from build123d import *

# Parameters (mm, degrees)
F1_DEPTH = 76.2
F2_R     = 12.7
F3_DEPTH = 25.4
F5_DEPTH = 25.4
F6_R     = 38.1
F7_R     = 38.1
F8_R     = 19.629033
F8_R_2   = 12.7
F9_DEPTH = 6.35


with BuildPart() as f1:
    # F0 (on Front) → F1 (new body, symmetric)
    with BuildSketch(Plane.XZ):
        Polygon((-76.2, 0), (0, 0), (0, 152.4), (-25.4, 152.4), (-25.4, 25.4), (-76.2, 25.4), align=None)
    extrude(amount=F1_DEPTH, both=True)

    # F2 (on face) → F3 (cut)
    with BuildSketch(Plane.YZ):
        with Locations((0, 101.6)):
            Circle(F2_R)
    extrude(amount=-F3_DEPTH, mode=Mode.SUBTRACT)

    # F4 (on face) → F5 (cut)
    with BuildSketch(Plane(origin=(0, 0, 0), x_dir=(1, 0, 0), z_dir=(0, 0, -1))):
        with BuildLine():
            ThreePointArc((-63.500749, -6.349625), (-69.781771, 0), (-63.500749, 6.349625))
            Line((-63.500749, 6.349625), (-76.2, 6.211669))
            Line((-76.2, 6.211669), (-76.2, -6.211669))
            Line((-76.2, -6.211669), (-63.500749, -6.349625))
        make_face()
        with BuildLine():
            ThreePointArc((-63.500749, -6.349625), (-58.966097, -4.51445), (-57.081771, 0))
            ThreePointArc((-57.081771, 0), (-58.966097, 4.51445), (-63.500749, 6.349625))
            ThreePointArc((-63.500749, 6.349625), (-69.781771, 0), (-63.500749, -6.349625))
        make_face()
    extrude(amount=-F5_DEPTH, mode=Mode.SUBTRACT)

    # F6
    f6_edges = [f1.edges().sort_by_distance(p)[0] for p in [
        (-12.7, -76.2, 152.4),
    ]]
    fillet(f6_edges, radius=F6_R)

    # F7
    f7_edges = [f1.edges().sort_by_distance(p)[0] for p in [
        (-12.7, 76.2, 152.4),
    ]]
    fillet(f7_edges, radius=F7_R)

    # F8 (on face) → F9 (cut)
    with BuildSketch(Plane(origin=(-25.4, 0, 0), x_dir=(0, -1, 0), z_dir=(-1, 0, 0))):
        with Locations((0, 101.6)):
            Circle(F8_R)
        with Locations((0, 101.6)):
            Circle(F8_R_2, mode=Mode.SUBTRACT)
    extrude(amount=-F9_DEPTH, mode=Mode.SUBTRACT)


solid = f1.part
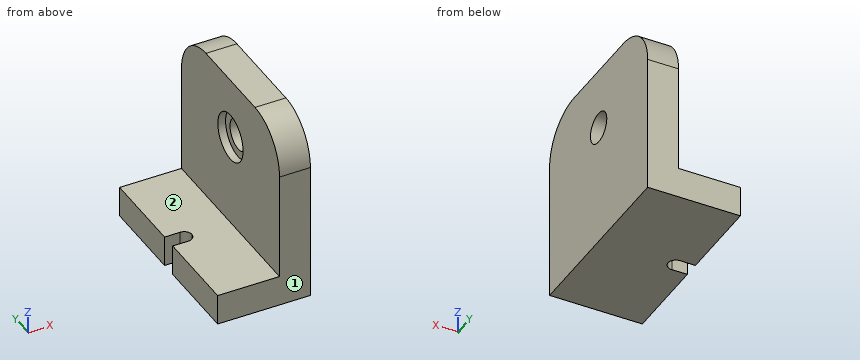
Geometry: final body of the model. Coordinates: model frame, mm. Face numbers are marked on the shaded views. A direction names the side the tool comes from. Give positions to 0.01 mm unless a question says otherwise; leave off trailing zeros. Write each loop counter-clockwise with the first axis right and the second up, starting at its lowest first coordinate (ties: lowest second). Pieces come first, ordered by that corner, then holes. Notation, with made-up numbers: (-20.75, 75.25) - (20.25, 75.25) arc R14 ccw to (20.25, 80.25) - close; hole circle Ø1 at (70, -1). An arc over 180 degrees is marked (long way). Return JSON: item names as keys, results as strings. Group by question number.
1) Section C-C on z = 66.5. Return the cut outline in (x, y).
2) Section D-D on x = -41.5. Return the cut outline in (y, z).
3) Set-up query: the marked faces 1 and 2. Return all of +Z, -Z, +X, -X, +Y, -Y with unobstructed straight access to the full face (end or side cutting, diameter ignored); none if empty.
4) First-contact query: P1, Ø15, axis at x = -39, y = 34.5, coming from the +Z side. Flat tip, straight axial feed; report the tip coordinate or a pass-through.
5) Section A-A on z = 101.6. Return the cut outline in (x, y), plus the area to 3 significant figures.
6) Line query: line 1 (Y direction, x = -14, z = 101); line 2 (Z direction, x = -21, y = 0); line 3 (Z direction, x = -9, y = 0). Output: solid intervals per line, ascending.
7) Section B-B on y = -36. Return the cut outline in (x, z), plus the area to 3 significant figures.
Filled in:
{
 "1": {"outline": "(-25.4, -76.2) - (0, -76.2) - (0, 76.2) - (-25.4, 76.2) - close"},
 "2": {"outline": "(-76.2, 0) - (76.2, 0) - (76.2, 25.4) - (-76.2, 25.4) - close"},
 "3": {"face 1": "+Z, -Z, +X, -X, -Y", "face 2": "+Z, -X, +Y, -Y"},
 "4": {"P1": "stops at z = 25.4"},
 "5": {"outline": "(-25.4, -76.2) - (0, -76.2) - (0, -12.7) - (-19.05, -12.7) - (-19.05, -19.63) - (-25.4, -19.63) - close; (-25.4, 19.63) - (-19.05, 19.63) - (-19.05, 12.7) - (0, 12.7) - (0, 76.2) - (-25.4, 76.2) - close", "area": "3,140 mm^2"},
 "6": {"line 1": "y = -76.2 to -12.69, 12.69 to 76.2", "line 2": "z = 0 to 81.97, 121.23 to 152.4", "line 3": "z = 0 to 88.9, 114.3 to 152.4"},
 "7": {"outline": "(-76.2, 0) - (0, 0) - (0, 152.4) - (-25.4, 152.4) - (-25.4, 25.4) - (-76.2, 25.4) - close", "area": "5,160 mm^2"}
}
